Work out the finished part from the listing and answer in its coordinate system (mm). Face numbers are marked on the shaded views. A direction names the side the tool comes from. Coordinates: 2 decimals unless noted, no trailing zeros. Write each loop counter-clockwise with the first axis right and the second up, starting at its lowest first coordinate (ties: lowest second). Pieces come first, ordered by that corner, then holes. Notation, with made-up numbers: M -25.5,78.5 L 12.5,78.5 A13 ccw 12.5,94.5 Z; hole C 46.5,87.5 d5. An arc over 180 degrees is marked long. Use CSV: the item, a comma, the result in double quotes.
from build123d import *

# Parameters (mm, degrees)
SKETCH1_W           = 14
SKETCH1_H           = 20
BOSS_EXTRUDE1_DEPTH = 10
SKETCH2_W           = 10
SKETCH2_H           = 10
BOSS_EXTRUDE2_DEPTH = 10
BOSS_EXTRUDE3_DEPTH = 5


with BuildPart() as part:
    # Sketch1 → Boss-Extrude1 (new body)
    with BuildSketch(Plane(origin=(0, 0, 0), x_dir=(1, 0, 0), z_dir=(0, 1, 0))):
        with Locations((7, 10)):
            Rectangle(SKETCH1_W, SKETCH1_H)
    extrude(amount=BOSS_EXTRUDE1_DEPTH)

    # Sketch2 → Boss-Extrude2 (add)
    with BuildSketch(Plane(origin=(0, 10, 0), x_dir=(1, 0, 0), z_dir=(0, 1, 0))):
        with Locations((7, 10)):
            Rectangle(SKETCH2_W, SKETCH2_H)
    extrude(amount=BOSS_EXTRUDE2_DEPTH)

    # Sketch3 → Boss-Extrude3 (add, symmetric)
    with BuildSketch(Plane(origin=(7, 0, 0), x_dir=(0, 0, -1), z_dir=(1, 0, 0))):
        with BuildLine():
            Line((1.25, 22), (1.25, 40.5))
            ThreePointArc((1.25, 40.5), (1.835786438, 41.914213562), (3.25, 42.5))
            Line((3.25, 42.5), (16.75, 42.5))
            ThreePointArc((16.75, 42.5), (18.164213562, 41.914213562), (18.75, 40.5))
            Line((18.75, 40.5), (18.75, 22))
            ThreePointArc((18.75, 22), (18.164213562, 20.585786438), (16.75, 20))
            Line((16.75, 20), (3.25, 20))
            ThreePointArc((3.25, 20), (1.835786438, 20.585786438), (1.25, 22))
        make_face()
    extrude(amount=BOSS_EXTRUDE3_DEPTH, both=True)


solid = part.part
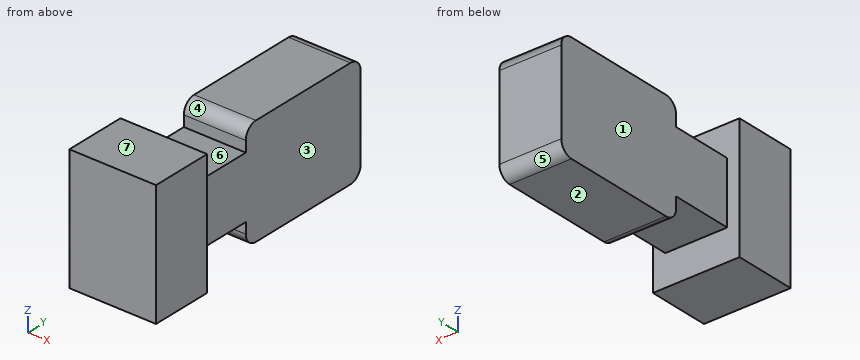
Item 1: Given pin 1 (8 mm diameter, centred on x = 7.5, y = 12.5, fed in from -Z); pin 2 (4 mm diameter, centred on x = 8.5, y = 35, fed in from -Z); pin 3 (10 mm diameter, centred on y = 31, z = -14, fed in from -X); pin 4 (4 mm diameter, centred on x = 10.5, y = 33, fed in from +Z), each flat-ended and moving along its own axis, determine where each tip first touches the part or whether it passes through.
Answer:
pin 1,"stops at z = -20"
pin 2,"stops at z = -18.75"
pin 3,"stops at x = 2"
pin 4,"stops at z = -1.25"
Item 2: The part is cut by section C-C (z = -7.75). Write down the section's boundary in (x, y).
Answer:
outline,"M 0,0 L 14,0 L 14,10 L 12,10 L 12,42.5 L 2,42.5 L 2,10 L 0,10 Z"
Item 3: The part is cut by section B-B (z = -2). Write down the section's boundary in (x, y).
Answer:
outline,"M 0,0 L 14,0 L 14,10 L 0,10 Z; M 2,20.44 L 12,20.44 L 12,42.06 L 2,42.06 Z"
Item 4: Consider probe 1 along Y at (x, z) = (2.5, -3.75); probe 2 along Y at (x, z) = (12.5, -2); probe 3 along X at (y, z) = (11.5, -8.25). Determine where each line is inside the solid, lowest interval first.
Answer:
probe 1,"y = 0 to 10, 20 to 42.5"
probe 2,"y = 0 to 10"
probe 3,"x = 2 to 12"
Item 5: The part is cut by section D-D (y = 13). Write down the section's boundary in (x, z), then the cut area to 3 significant figures.
Answer:
outline,"M 2,-15 L 12,-15 L 12,-5 L 2,-5 Z"
area,"100 mm2"
Item 6: The part is cut by section A-A (x = 10.75). Write down the section's boundary in (y, z).
Answer:
outline,"M 0,-20 L 10,-20 L 10,-15 L 20,-15 L 20,-16.75 A2 ccw 22,-18.75 L 40.5,-18.75 A2 ccw 42.5,-16.75 L 42.5,-3.25 A2 ccw 40.5,-1.25 L 22,-1.25 A2 ccw 20,-3.25 L 20,-5 L 10,-5 L 10,0 L 0,0 Z"
Item 7: A tool of negligible diameter and unlimited length cuts with its end or side. For the marked faces 1, 2 and 3, from which of +Z, -Z, +X, -X, +Y, -Y can it reach the whole face along a straight path? Write none if from no direction.
Answer:
face 1,"+Z, -Z, -X, +Y"
face 2,"-Z, +X, -X, +Y"
face 3,"+Z, -Z, +X, +Y"
Item 8: For a pull along Y with two mould halves and no side action, classify the marked faces 4, 5, 6 and 7 as released by +Y, released by -Y, zero draft, split by the parting line, or undercut.
Answer:
face 4,"undercut"
face 5,"released by +Y"
face 6,"undercut"
face 7,"zero draft"
